Verification items for this drawing (mm, ordinates from the low corner). Coordinates: 2 decimals unless noted, no trailing zeros. Write each loop counter-clockwise with the first axis right and the second up, starting at its lowest first coordinate (ties: lowest second). Pieces come first, ordered by that corner, then holes. Notation, with made-up numbers: (81.25, 43) -> (99.25, 43) arc R7 ccw to (99.25, 52) -> close; hole circle Ø8 at (36, 69). An arc over 180 degrees is marked (long way). Answer as CSV lines item,"result".
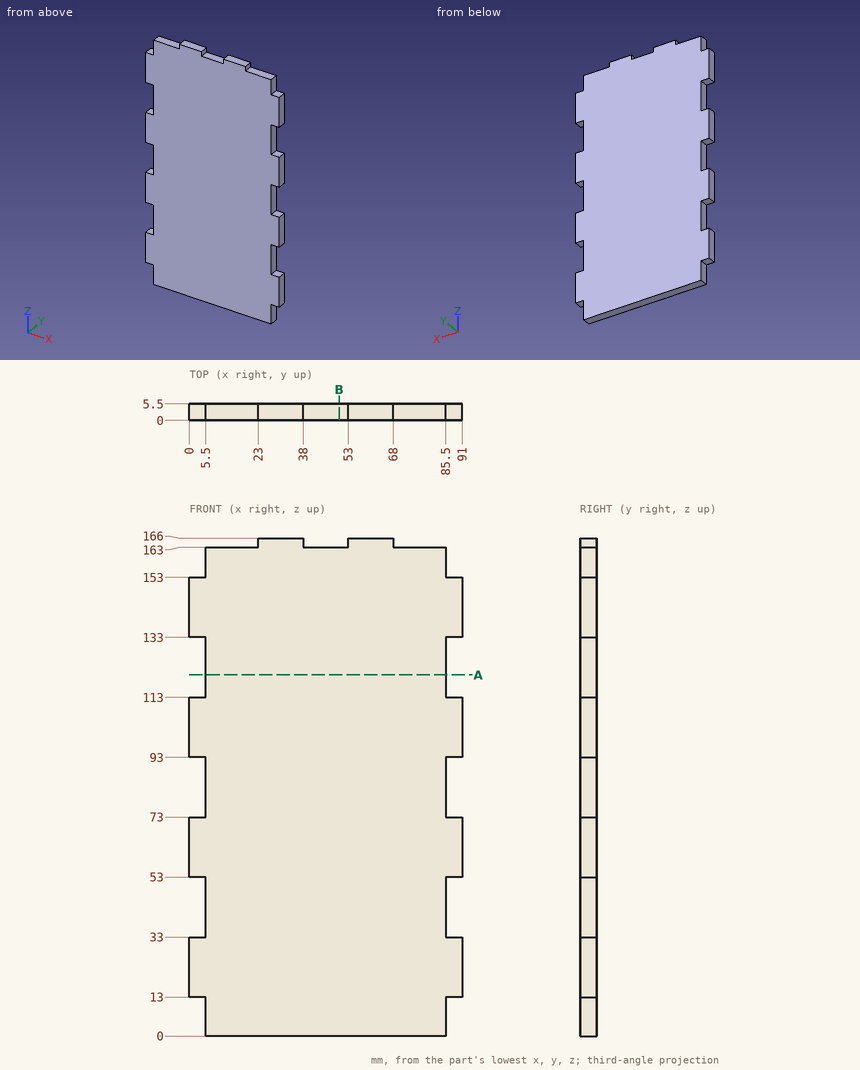
Item 1: Cross-section at A-A, the plane z = 120.5. Record the cut outline in (x, y), plus the area to 3 significant figures.
Responses:
outline,"(5.5, 0) -> (85.5, 0) -> (85.5, 5.5) -> (5.5, 5.5) -> close"
area,"440 mm2"
Item 2: Cross-section at B-B, the plane x = 50. Record the cut outline in (y, z), plus the area to 4 significant figures.
Responses:
outline,"(0, 0) -> (5.5, 0) -> (5.5, 163) -> (0, 163) -> close"
area,"896.5 mm2"
Item 3: Thickness scan on probe 1 along Z at (x, y) = (4, 2.1); probe 2 along Z at (x, y) = (80.5, 0.35); probe 3 along X at (y, z) = (2.95, 75.5). Record the ranges inside material, lowest first.
Responses:
probe 1,"z = 13 to 33, 53 to 73, 93 to 113, 133 to 153"
probe 2,"z = 0 to 163"
probe 3,"x = 5.5 to 85.5"
Item 4: Depth check by flat-ended pin: pin 1 Ø1.6 at (x, y) = (2, 2) entering from -Z; pin 2 Ø1.6 at (x, y) = (3.5, 1.5) entering from +Z; pin 3 Ø2 at (y, z) = (3, 42) entering from +X. Enter the tip coordinate at first touch or a pass-through.
Responses:
pin 1,"stops at z = 13"
pin 2,"stops at z = 153"
pin 3,"stops at x = 85.5"
